from build123d import *

# Parameters (mm, degrees)
SKETCH_1_W      = 30
SKETCH_1_H      = 30
SKETCH_1_R      = 8
EXTRUDE_1_DEPTH = 697.8
SKETCH_2_W      = 10
SKETCH_2_H      = 3.2
EXTRUDE_2_DEPTH = 14.4


with BuildPart() as part:
    # 草图1 → 凸台-拉伸1 (new body)
    with BuildSketch(Plane.XY):
        Rectangle(SKETCH_1_W, SKETCH_1_H)
        Circle(SKETCH_1_R, mode=Mode.SUBTRACT)
    extrude(amount=EXTRUDE_1_DEPTH)

    # 草图2 → 凸台-拉伸2 (add)
    with BuildSketch(Plane.XY.offset(697.8)):
        with Locations((0, 16.6)):
            Rectangle(SKETCH_2_W, SKETCH_2_H)
    extrude_2 = extrude(amount=-EXTRUDE_2_DEPTH)

    # 镜向1: 凸台-拉伸2 across plane
    add(extrude_2.mirror(Plane.XY.offset(348.9)))


solid = part.part
Geometry: final body of the model. Coordinates: model frame, mm. Round coordinates to 2 decimals unless told otherwise and drop trailing zeros. Loops run counter-clockwise (first coordinate to the right, second up) from the corner with the lowest first, then second, coordinate; pieces in that order, holes last. Notation, with made-up numbers: (78, 74) - (129, 74) arc R29 cw to (129, 98) - close; hole circle Ø9 at (-21.5, 32). An arc over 180 degrees is marked (long way). Write each question's results on one line, items separated by ' | '. Start each with the question number.
1) Mould query, pull axis Y, two halves, no side actions, for faces 1 (the face through (0, -15, 344)), 2 (the face through (15, 0, 344)), 3 (the face through (-1.73, -7.81, 344.02)). Classes: released by +Y, released by -Y, zero draft, split by the parting line, or undercut.
2) Cut plane A-A on x = 0. Return loops of the section in (y, z).
3) First-contact query: P1, Ø3.5, axis at x = 1, y = 16, coming from the -Z side; P2, Ø1.6, axis at y = 17, z = 690, coming from the -X side; P3, Ø9, axis at x = 2.5, z = 189, coming from the +Y side; P4, Ø2.5, axis at y = 17, z = 9.5, coming from the +X side. Flat tips, straight axial feed; report the tip coordinate or a pass-through.
4) Cut plane C-C on z = 249. Return loops of the section in (x, y).
5) Line query: probe 1 along Y at (x, z) = (0, 445); probe 2 along Y at (x, z) = (-1.25, 195); probe 3 along Y at (x, z) = (-12.5, 614.5). Output: solid intervals per line, ascending. Write a range as [from, to].
6) Cut plane B-B on y = 0. Return loops of the section in (x, z), then the cut area to 3 significant figures.
Verdict:
1) face 1: released by -Y | face 2: zero draft | face 3: undercut
2) outline: (-15, 0) - (-8, 0) - (-8, 697.8) - (-15, 697.8) - close; (8, 0) - (18.2, 0) - (18.2, 14.4) - (15, 14.4) - (15, 683.4) - (18.2, 683.4) - (18.2, 697.8) - (8, 697.8) - close
3) P1: stops at z = 0 | P2: stops at x = -5 | P3: stops at y = 15 | P4: stops at x = 5
4) outline: (-15, -15) - (15, -15) - (15, 15) - (-15, 15) - close; hole circle Ø16 at (0, 0)
5) probe 1: y = [-15, -8], [8, 15] | probe 2: y = [-15, -7.9], [7.9, 15] | probe 3: y = [-15, 15]
6) outline: (-15, 0) - (-8, 0) - (-8, 697.8) - (-15, 697.8) - close; (8, 0) - (15, 0) - (15, 697.8) - (8, 697.8) - close | area: 9,770 mm2
